For this review, use the dimensioned drawing (mm, ordinates from the lowest corner) and the shaded views. Round coordinates to 2 decimals unless told otherwise and drop trailing zeros. Write each loop counter-clockwise with the first axis right and the second up, starting at its lowest first coordinate (ties: lowest second). Pieces come first, ordered by that corner, then holes. Notation, with made-up numbers: (-38, 77) - (-19, 77) arc R8 cw to (-19, 89) - close; hole circle Ø1 at (68, 39). An arc over 180 degrees is marked (long way). Write each question's results on one line, items separated by ' | '.
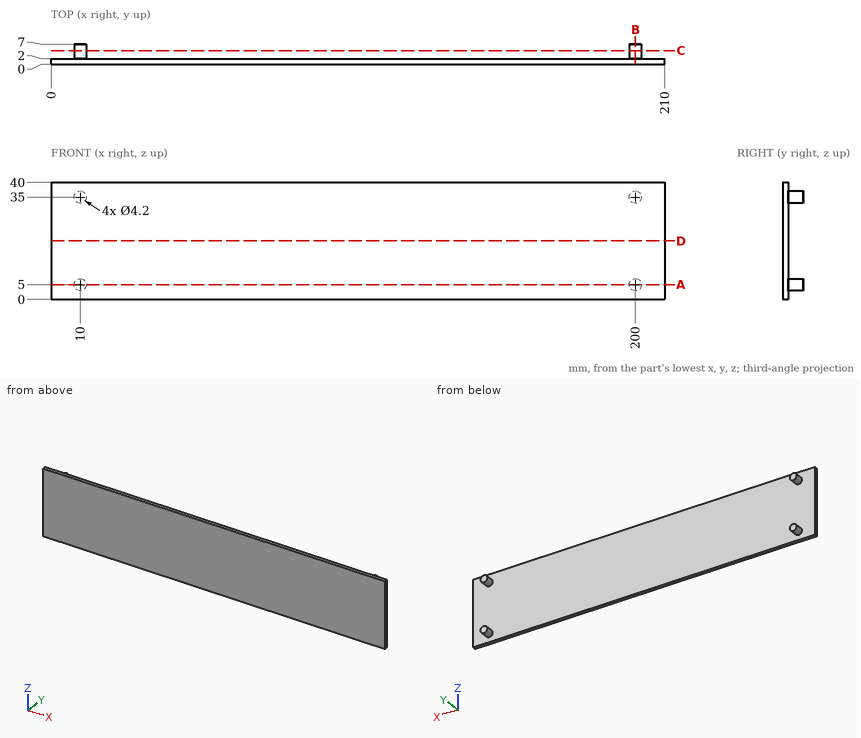
Q1. We need section D-D (z = 20). State the section outline as (x, y) points.
Evaluation:
outline: (0, 0) - (210, 0) - (210, 2) - (0, 2) - close
Q2. We need section A-A (z = 5). State the section outline as (x, y) points.
Evaluation:
outline: (0, 0) - (210, 0) - (210, 2) - (202.1, 2) - (202.1, 7) - (197.9, 7) - (197.9, 2) - (12.1, 2) - (12.1, 7) - (7.9, 7) - (7.9, 2) - (0, 2) - close
Q3. For probe 1 along Y at (x, z) = (43.5, 4.5); probe 2 along X at (y, z) = (2.25, 4.5); probe 3 along X at (y, z) = (5, 34), list the stretches that pass through material, from the lowest coordinate up.
Evaluation:
probe 1: y = 0 to 2 | probe 2: x = 7.96 to 12.04, 197.96 to 202.04 | probe 3: x = 8.15 to 11.85, 198.15 to 201.85
Q4. We need section C-C (y = 4.75). State the section outline as (x, z) points, plus the area to 3 significant figures.
Evaluation:
outline: circle Ø4.2 at (10, 5); circle Ø4.2 at (10, 35); circle Ø4.2 at (200, 5); circle Ø4.2 at (200, 35) | area: 55.4 mm^2
Q5. We need section B-B (x = 200). State the section outline as (y, z) points, plus the area to 3 significant figures.
Evaluation:
outline: (0, 0) - (2, 0) - (2, 2.9) - (7, 2.9) - (7, 7.1) - (2, 7.1) - (2, 32.9) - (7, 32.9) - (7, 37.1) - (2, 37.1) - (2, 40) - (0, 40) - close | area: 122 mm^2
Q6. Insertion check: P1, Ø10, axis at x = 184, z = 27.5, coming from the +Y side. The pin has a flat end and moves straight along its axis. Give the tip position at first contact, or say it passes through.
Evaluation:
P1: stops at y = 2
